Geometry check sheet. Reference: the model listing, model coordinates, mm. Face numbers are marked on the shaded views. A direction names the side the tool comes from. Round coordinates to 2 decimals unless told otherwise and drop trailing zeros. Loops run counter-clockwise (first coordinate to the right, second up) from the corner with the lowest first, then second, coordinate; pieces in that order, holes last. Notation, with made-up numbers: M -1.5,45.5 L 4.5,45.5 A29 cw 4.5,79.5 Z; hole C -10.5,45.25 d10. An arc over 180 degrees is marked long. Answer in a Markdown table with one row per item. Add a question column.
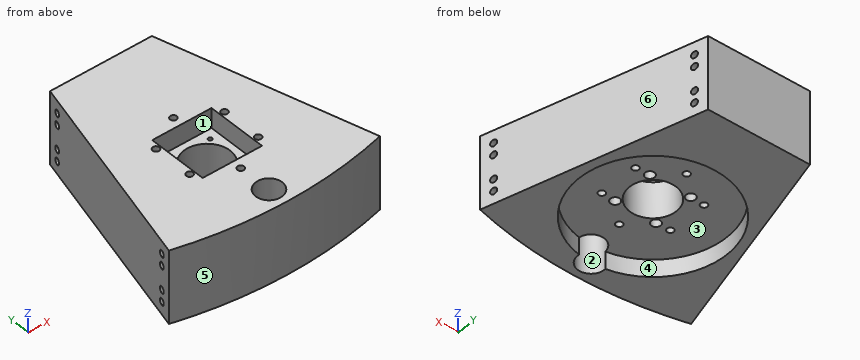
Autodesk Inventor part; units mm, degrees
ref_plane "YZ Plane" through (0, 0, 0) normal (1, 0, 0) x (0, 1, 0)
ref_plane "XZ Plane" through (0, 0, 0) normal (0, 1, 0) x (-1, 0, 0)
ref_plane "XY Plane" through (0, 0, 0) normal (0, 0, 1) x (1, 0, 0)
sketch "Sketch1" plane through (0, 0, 0) normal (0, 0, 1) x (1, 0, 0)
  line L0 (0, 0) -> (160, 0)
  line L1 (160, 0) -> (118.589, 154.5481)
  line L2 (41.411, 154.5481) -> (0, 0)
  line L3 (41.411, 154.5481) -> (118.589, 154.5481)
  dimension "d0" = 160
  dimension "d1" = 160
  dimension "d2" = 75
  dimension "d8" = 75
extrude "Extrusion1" add sketch "Sketch1" along normal blind 55
sketch "Sketch7" plane through (0, 0, 0) normal (0, 0, -1) x (-1, 0, 0)
  circle A0 centre (-80, 304.672) radius 315 construction
  line L0 (0, 0) -> (-160, 0)
  arc A1 (-160, 0) -> (0, 0) centre (-80, 304.672) ccw
  dimension "d28" = 630
extrude "Extrusion6" add sketch "Sketch7" against normal blind 55
sketch "Sketch19" plane through (0, 0, 0) normal (0, 0, -1) x (-1, 0, 0)
  circle A0 centre (-80, 60) radius 55
  line L0 (-118.589, 154.5481) -> (-41.411, 154.5481)
  point P0 (0, 0)
  point P1 (-80, 154.5481)
  dimension "d112" = 110
  dimension "d113" = 60
extrude "Extrusion19" cut sketch "Sketch19" against normal blind 13
sketch "Sketch20" plane through (80, 60, 13) normal (0, 0, -1) x (-1, 0, 0)
  circle A0 centre (0, 0) radius 55 construction
  circle A1 centre (0, 0) radius 17.5
  point P0 (80, -60)
  dimension "d116" = 35
extrude "Extrusion20" cut sketch "Sketch20" against normal through all
sketch "Sketch21" plane through (0, 0, 55) normal (0, 0, 1) x (1, 0, 0)
  circle A0 centre (80, 60) radius 17.5 construction
  line L0 (57.5, 37.5) -> (102.5, 37.5)
  line L1 (102.5, 37.5) -> (102.5, 82.5)
  line L2 (102.5, 82.5) -> (57.5, 82.5)
  line L3 (57.5, 82.5) -> (57.5, 37.5)
  point P0 (0, 0)
  point P1 (57.5, 60)
  point P2 (80, 82.5)
  dimension "d119" = 45
  dimension "d120" = 45
extrude "Extrusion21" cut sketch "Sketch21" against normal blind 15
sketch "Sketch23" plane through (0, 0, 40) normal (0, 0, 1) x (1, 0, 0)
  line L0 (64.5, 75.5) -> (95.5, 75.5) construction
  line L1 (95.5, 75.5) -> (95.5, 44.5) construction
  line L2 (95.5, 44.5) -> (64.5, 44.5) construction
  line L3 (64.5, 44.5) -> (64.5, 75.5) construction
  circle A0 centre (80, 60) radius 17.5 construction
  circle A1 centre (95.5, 75.5) radius 1.5
  circle A2 centre (95.5, 44.5) radius 1.5
  circle A3 centre (64.5, 44.5) radius 1.5
  circle A4 centre (64.5, 75.5) radius 1.5
  point P0 (0, 0)
  point P1 (64.5, 60)
  point P2 (80, 75.5)
  dimension "d126" = 31
  dimension "d127" = 31
  dimension "d128" = 3
  dimension "d129" = 3
  dimension "d130" = 3
  dimension "d131" = 3
extrude "Extrusion23" cut sketch "Sketch23" against normal through all
sketch "Sketch25" plane through (80, 60, 13) normal (0, 0, -1) x (-1, 0, 0)
  circle A0 centre (0, 30) radius 2.5
  circle A1 centre (0, 0) radius 55 construction
  circle A2 centre (-25.9808, 15) radius 2.5
  circle A3 centre (-25.9808, -15) radius 2.5
  circle A4 centre (0, -30) radius 2.5
  circle A5 centre (25.9808, -15) radius 2.5
  circle A6 centre (25.9808, 15) radius 2.5
  point P0 (80, -60)
  dimension "d138" = 5
  dimension "d139" = 30
  dimension "d142" = 360
extrude "Extrusion25" cut sketch "Sketch25" against normal through all
sketch "Sketch26" plane through (80, 60, 13) normal (0, 0, -1) x (-1, 0, 0)
  circle A0 centre (15.5, -15.5) radius 1.5
  circle A1 centre (-15.5, -15.5) radius 1.5
  circle A2 centre (-15.5, 15.5) radius 1.5
  circle A3 centre (15.5, 15.5) radius 1.5
  circle A4 centre (15.5, -15.5) radius 3.5
  circle A5 centre (-15.5, -15.5) radius 1.5
  circle A6 centre (-15.5, -15.5) radius 3.5
  circle A7 centre (-15.5, 15.5) radius 3.5
  circle A8 centre (15.5, 15.5) radius 3.5
  point P0 (80, -60)
  dimension "d146" = 7
  dimension "d147" = 7
  dimension "d148" = 7
  dimension "d149" = 7
extrude "Extrusion26" cut sketch "Sketch26" against normal blind 20 contours A0 | A1 | A2 | A3 | A4 | A6 | A7 | A8
sketch "Sketch27" plane through (0, 0, 55) normal (0, 0, 1) x (1, 0, 0)
  circle A0 centre (80, 4.836) radius 10
  line L0 (118.589, 154.5481) -> (41.411, 154.5481) construction
  line L1 (80, 154.5481) -> (80, -10.328) construction
  arc A1 (0, 0) -> (160, 0) centre (80, 304.672) ccw construction
  dimension "d152" = 20
  dimension "d153" = 15.164
extrude "Extrusion27" cut sketch "Sketch27" against normal through all
sketch "Sketch28" plane through (41.411, 154.5481, 0) normal (-0.9659, 0.2588, 0) x (0, 0, 1)
  line L0 (9.525, -150.46) -> (9.525, -9.54) construction
  circle A0 centre (9.525, -150.46) radius 2.5
  circle A1 centre (9.525, -9.54) radius 2.5
  line L1 (0, 0) -> (0, -160)
  circle A2 centre (18.4199, -9.54) radius 2.5
  circle A3 centre (36.5801, -9.54) radius 2.5
  circle A4 centre (45.475, -9.54) radius 2.5
  line L2 (55, 0) -> (55, -160)
  circle A5 centre (18.4199, -150.46) radius 2.5
  circle A6 centre (36.5801, -150.46) radius 2.5
  circle A7 centre (45.475, -150.46) radius 2.5
  point P0 (9.525, -80)
  point P1 (0, -80)
  dimension "d156" = 140.92
  dimension "d157" = 5
  dimension "d158" = 5
  dimension "d159" = 9.525
  dimension "d160" = 5
  dimension "d161" = 5
  dimension "d162" = 5
  dimension "d163" = 18.4199
  dimension "d164" = 18.4199
  dimension "d165" = 9.525
  dimension "d166" = 5
  dimension "d167" = 5
  dimension "d168" = 5
extrude "Extrusion28" cut sketch "Sketch28" against normal blind 25
sketch "Sketch29" plane through (118.589, 154.5481, 55) normal (0.9659, 0.2588, 0) x (0, 0, -1)
  line L0 (9.525, -150.46) -> (9.525, -9.54) construction
  circle A0 centre (9.525, -150.46) radius 2.5
  circle A1 centre (9.525, -9.54) radius 2.5
  circle A2 centre (18.4199, -9.54) radius 2.5
  circle A3 centre (36.5801, -9.54) radius 2.5
  circle A4 centre (45.475, -9.54) radius 2.5
  circle A5 centre (18.4199, -150.46) radius 2.5
  circle A6 centre (36.5801, -150.46) radius 2.5
  circle A7 centre (45.475, -150.46) radius 2.5
  line L1 (0, -160) -> (0, 0)
  line L2 (55, -160) -> (55, 0)
  point P0 (9.525, -80)
  point P1 (0, -80)
  point P2 (0, -80)
  dimension "d169" = 140.92
  dimension "d170" = 5
  dimension "d171" = 5
  dimension "d173" = 5
  dimension "d174" = 5
  dimension "d175" = 5
  dimension "d179" = 5
  dimension "d180" = 5
  dimension "d181" = 5
  dimension "d184" = 9.525
  dimension "d185" = 18.4199
  dimension "d186" = 9.525
  dimension "d187" = 18.4199
extrude "Extrusion29" cut sketch "Sketch29" against normal blind 25
properties part number "CA001" material "ABS Plastic"
1) Cross-section at D-D, the plane y = 111. Record the boundary of the cut face in (x, z).
2) Cross-section at A-A, the plane x = 80. Record the boundary of the cut face in (y, z).
3) Set-up check for the marked faces 1, 2 and 3: record each of +Z, -Z, +X, -X, +Y, -Y from which the full face is reachable in a straight line by a thin tool's end or side.
4) Draft check along X on the marked faces 4, 5 and 6. Enter one of: +X half, -X half, draft (parallel to the pull), parting line (faces both ways), or undercut.
5) Cross-section at C-C, the plane z = 37. Count the separate pieces of the cut face and the enclosed holes in it, plus the area to 3 significant figures.
6) Thickness scan on L1, parallel to Y at x = 107, z = 33.5; L2, parallel to Y at x = 80, z = 29; L3, parallel to Y at x = 65.5, z = 38. Record the ranges inside material, lowest first. Write a range as [from, to].
7) Go/stop test with flat-tipped pins: pin 1 (1.5 mm diameter, centred on y = 29, z = 19, fed in from +X); pin 2 (4.5 mm diameter, centred on x = 87.5, z = 49.5, fed in from -Y); pin 3 (3.5 mm diameter, centred on x = 96.5, y = 44.5, fed in from -Z). Record where each tip stops, or that it passes through.
8) Cross-section at B-B, the plane y = 62. Record the boundary of the cut face in (x, z).
Worked answers:
| question | item | result |
|---|---|---|
| 1 | outline | M 29.74,0 L 59.41,0 L 59.41,13 L 100.59,13 L 100.59,0 L 130.26,0 L 130.26,55 L 29.74,55 Z |
| 2 | outline | M -10.33,0 L -5.16,0 L -5.16,55 L -10.33,55 Z; M 14.84,13 L 27.5,13 L 27.5,55 L 14.84,55 Z; M 32.5,13 L 42.5,13 L 42.5,40 L 37.5,40 L 37.5,55 L 32.5,55 Z; M 77.5,13 L 87.5,13 L 87.5,55 L 82.5,55 L 82.5,40 L 77.5,40 Z; M 92.5,13 L 115,13 L 115,0 L 154.55,0 L 154.55,55 L 92.5,55 Z |
| 3 | face 1 | +Z |
| 3 | face 2 | +Z, -Z |
| 3 | face 3 | -Z |
| 4 | face 4 | undercut |
| 4 | face 5 | parting line |
| 4 | face 6 | +X half |
| 5 | separate pieces | 1 |
| 5 | enclosed holes | 12 |
| 5 | area | 17,500 mm2 |
| 6 | L1 | y = [-9.17, 42.72], [47.28, 72.72], [77.28, 154.55] |
| 6 | L2 | y = [-10.33, -5.16], [14.84, 27.5], [32.5, 42.5], [77.5, 87.5], [92.5, 154.55] |
| 6 | L3 | y = [-9.99, 43.38], [45.62, 50.2], [69.8, 74.38], [76.62, 154.55] |
| 7 | pin 1 | stops at x = 152.43 |
| 7 | pin 2 | stops at y = -10.28 |
| 7 | pin 3 | stops at z = 33 |
| 8 | outline | M 16.61,0 L 25.04,0 L 25.04,13 L 62.61,13 L 62.61,40 L 57.5,40 L 57.5,55 L 16.61,55 Z; M 97.39,13 L 134.96,13 L 134.96,0 L 143.39,0 L 143.39,55 L 102.5,55 L 102.5,40 L 97.39,40 Z |
